Can you work these out from the model? Positions are in its coordinate system, mm. Give positions to 0.01 mm unless a question says otherwise; leave off trailing zeros. Loops run counter-clockwise (first coordinate to the right, second up) from the corner with the lowest first, then second, coordinate; pieces in that order, holes last.
from build123d import *

# Parameters (mm, degrees)
SKETCH1_W                   = 88
SKETCH1_H                   = 211
BOSS_EXTRUDE1_DEPTH         = 2
CUT_EXTRUDE2_DEPTH          = 2
SKETCH4_R                   = 5
CUT_EXTRUDE3_DEPTH          = 3
FILLET2_R                   = 3
SKETCH23_W                  = 2
SKETCH23_H                  = 211
SKETCH23_W_2                = 2.150374681
CUT_EXTRUDE5_DEPTH          = 10
SKETCH29_W                  = 5.911493913
SKETCH29_H                  = 211
SKETCH29_W_2                = 4.036537762
CUT_EXTRUDE10_DEPTH         = 2
F_3_0MM_DOWEL_HOLE1_D       = 3
TAP_DRILL_FOR_M3X0_5_TAP1_D = 2.5


with BuildPart() as part:
    # Sketch1 → Boss-Extrude1 (new body)
    with BuildSketch(Plane.XY):
        with Locations((44, 105.5)):
            Rectangle(SKETCH1_W, SKETCH1_H)
    extrude(amount=BOSS_EXTRUDE1_DEPTH)

    # Sketch3 → Cut-Extrude2 (cut)
    with BuildSketch(Plane.XY.offset(2)):
        Polygon((73, 133.88804004), (50, 147.167096231), (50, 115.5), (73, 115.5), align=None)
        Polygon((38, 115.5), (38, 147.167096231), (15, 133.88804004), (15, 115.5), align=None)
        Polygon((15, 143.125644347), (36, 155.25), (15, 167.374355653), align=None)
        Polygon((73, 143.125644347), (73, 167.374355653), (52, 155.25), align=None)
        Polygon((73, 196), (50, 196), (50, 163.332903769), (73, 176.61195996), align=None)
        Polygon((38, 163.332903769), (38, 196), (15, 196), (15, 176.61195996), align=None)
    cut_extrude2 = extrude(amount=-CUT_EXTRUDE2_DEPTH, mode=Mode.SUBTRACT)

    # Sketch4 → Cut-Extrude3 (cut, through all)
    with BuildSketch(Plane.XY.offset(2)):
        with Locations((44, 155.25)):
            Circle(SKETCH4_R)
    cut_extrude3 = extrude(amount=-CUT_EXTRUDE3_DEPTH, mode=Mode.SUBTRACT)

    # Mirror2: Cut-Extrude2, Cut-Extrude3 across plane
    add(cut_extrude2.mirror(Plane.ZX.offset(105.5)), mode=Mode.SUBTRACT)
    add(cut_extrude3.mirror(Plane.ZX.offset(105.5)), mode=Mode.SUBTRACT)

    # Fillet2
    fillet2_edges = [part.edges().sort_by_distance(p)[0] for p in [
        (36, 55.75, 1),
        (15, 43.625644347, 1),
        (15, 67.874355653, 1),
        (38, 95.5, 1),
        (38, 63.832903769, 1),
        (15, 77.11195996, 1),
        (15, 95.5, 1),
        (73, 15, 1),
        (50, 15, 1),
        (50, 47.667096231, 1),
        (73, 34.38804004, 1),
        (73, 43.625644347, 1),
        (52, 55.75, 1),
        (73, 67.874355653, 1),
        (15, 15, 1),
        (15, 34.38804004, 1),
        (38, 47.667096231, 1),
        (38, 15, 1),
        (73, 77.11195996, 1),
        (50, 63.832903769, 1),
        (50, 95.5, 1),
        (73, 95.5, 1),
        (15, 167.374355653, 1),
        (36, 155.25, 1),
        (15, 143.125644347, 1),
        (38, 147.167096231, 1),
        (38, 115.5, 1),
        (15, 115.5, 1),
        (15, 133.88804004, 1),
        (50, 196, 1),
        (73, 196, 1),
        (73, 176.61195996, 1),
        (50, 163.332903769, 1),
        (52, 155.25, 1),
        (73, 167.374355653, 1),
        (73, 143.125644347, 1),
        (15, 176.61195996, 1),
        (15, 196, 1),
        (38, 196, 1),
        (38, 163.332903769, 1),
        (50, 147.167096231, 1),
        (73, 133.88804004, 1),
        (73, 115.5, 1),
        (50, 115.5, 1),
    ]]
    fillet(fillet2_edges, radius=FILLET2_R)

    # Sketch23 → Cut-Extrude5 (cut)
    with BuildSketch(Plane.XY.offset(2)):
        with Locations((87, 105.5)):
            Rectangle(SKETCH23_W, SKETCH23_H)
        with Locations((1.075187341, 105.5)):
            Rectangle(SKETCH23_W_2, SKETCH23_H)
    extrude(amount=-CUT_EXTRUDE5_DEPTH, mode=Mode.SUBTRACT)

    # Sketch29 → Cut-Extrude10 (cut)
    with BuildSketch(Plane(origin=(0, 0, 0), x_dir=(-1, 0, 0), z_dir=(0, 0, -1))):
        with Locations((-1.044253043, 105.5)):
            Rectangle(SKETCH29_W, SKETCH29_H)
        with Locations((-86.018268881, 105.5)):
            Rectangle(SKETCH29_W_2, SKETCH29_H)
    extrude(amount=-CUT_EXTRUDE10_DEPTH, mode=Mode.SUBTRACT)

    # Ø3.0mm Dowel Hole1 (through all)
    with Locations(Plane.XY.offset(2)):
        with Locations((24, 205), (64, 205), (9, 184), (79, 184), (9, 135), (79, 135), (79, 109.2), (9, 109.2), (9, 79.2), (79, 79.2), (79, 59.2), (9, 59.2), (9, 33.2), (79, 33.2), (64, 6), (24, 6)):
            Hole(F_3_0MM_DOWEL_HOLE1_D / 2)

    # Tap Drill for M3x0.5 Tap1 (through all)
    with Locations(Plane.XY.offset(2)):
        with Locations((9, 23), (79, 23), (9, 196), (79, 196)):
            Hole(TAP_DRILL_FOR_M3X0_5_TAP1_D / 2)


solid = part.part
(1) Please list where these lines run through material, in increasing order: probe 1 along X at (y, z) = (184, 1.4); probe 2 along X at (y, z) = (205, 0.4); probe 3 along X at (y, z) = (120.5, 1.5).
Returned:
probe 1: x = 4 to 7.5, 10.5 to 15, 38 to 50, 73 to 77.5, 80.5 to 84
probe 2: x = 4 to 22.5, 25.5 to 62.5, 65.5 to 84
probe 3: x = 4 to 15, 38 to 50, 73 to 84
(2) Suppose I cut it at B-B on z = 1. Give the number of separate pieces and of enclosed holes in the cut face, plus the area to 3 significant figures.
Returned:
separate pieces: 1
enclosed holes: 34
area: 11,000 mm2
(3) Will this pin go through, and if not, where does the flat tip stop? P1, Ø4, axis at x = 9, y = 79.2, coming from the +Z side.
Returned:
P1: stops at z = 2
(4) Thinking about a two-plate mould opening in X: for faces 1 (the flat face through (43, 107, 2)), 2 (the flat face through (25.42, 61.86, 1.01)), which applies, pulls with the +X half, pulls with the -X half, needs draft (parallel to the pull), parting line crosses it, or undercut?
Returned:
face 1: needs draft
face 2: undercut
(5) Suppose I cut it at A-A on y = 155.25. List the corners of the cut face in (x, z) for me, plus the area to 3 significant figures.
Returned:
outline: (4, 0) - (15, 0) - (15, 2) - (4, 2) - close; (33, 0) - (39, 0) - (39, 2) - (33, 2) - close; (49, 0) - (55, 0) - (55, 2) - (49, 2) - close; (73, 0) - (84, 0) - (84, 2) - (73, 2) - close
area: 68.0 mm2
